from build123d import *

# Parameters (mm, degrees)
SKETCH_1_W             = 40
SKETCH_1_H             = 27
EXTRUDE_1_DEPTH        = 60
SKETCH_2_R             = 2.5
CUT_EXTRUDE_1_DEPTH    = 27
PATTERN_LINEAR_1_COUNT = 2
PATTERN_LINEAR_1_PITCH = 46
SKETCH_4_R             = 1.65
CUT_EXTRUDE_3_DEPTH    = 27
SKETCH_5_W             = 20
SKETCH_5_H             = 60
CUT_EXTRUDE_4_DEPTH    = 30
PATTERN_LINEAR_2_COUNT = 2
PATTERN_LINEAR_2_PITCH = 10


with BuildPart() as part:
    # Эскиз1 → Бобышка-Вытянуть1 (new body)
    with BuildSketch(Plane.XY):
        Rectangle(SKETCH_1_W, SKETCH_1_H)
    extrude(amount=EXTRUDE_1_DEPTH)

    # Эскиз2 → Вырез-Вытянуть1 (cut)
    with BuildSketch(Plane(origin=(0, 13.5, 0), x_dir=(1, 0, 0), z_dir=(0, 1, 0))):
        with Locations(Location((-10, -7, 0), (0, 0, 180))):
            Circle(SKETCH_2_R)
    cut_extrude_1 = extrude(amount=-CUT_EXTRUDE_1_DEPTH, mode=Mode.SUBTRACT)

    # Линейный массив1: Вырез-Вытянуть1 ×2
    with Locations(*[(0, 0, i * PATTERN_LINEAR_1_PITCH) for i in range(1, PATTERN_LINEAR_1_COUNT)]):
        add(cut_extrude_1, mode=Mode.SUBTRACT)

    # Эскиз4 → Вырез-Вытянуть3 (cut)
    with BuildSketch(Plane(origin=(0, 13.5, 0), x_dir=(1, 0, 0), z_dir=(0, 1, 0))):
        with Locations(Location((-15, -15, 0), (0, 0, 270))):
            Circle(SKETCH_4_R)
        with Locations(Location((-15, -45, 0), (0, 0, 270))):
            Circle(SKETCH_4_R)
    cut_extrude_3 = extrude(amount=-CUT_EXTRUDE_3_DEPTH, mode=Mode.SUBTRACT)

    # Эскиз5 → Вырез-Вытянуть4 (cut)
    with BuildSketch(Plane.XZ.offset(13.5)):
        with Locations((10, 30)):
            Rectangle(SKETCH_5_W, SKETCH_5_H)
    extrude(amount=-CUT_EXTRUDE_4_DEPTH, mode=Mode.SUBTRACT)

    # Линейный массив2: Вырез-Вытянуть3 ×2
    with Locations(*[(i * PATTERN_LINEAR_2_PITCH, 0, 0) for i in range(1, PATTERN_LINEAR_2_COUNT)]):
        add(cut_extrude_3, mode=Mode.SUBTRACT)


solid = part.part
Input: part model. Units: mm. Frame: model coordinates. Round coordinates to 2 decimals unless told otherwise and drop trailing zeros. Loops run counter-clockwise (first coordinate to the right, second up) from the corner with the lowest first, then second, coordinate; pieces in that order, holes last. Notation, with made-up numbers: (60.5, 80) -> (106.5, 80) arc R19 cw to (106.5, 110) -> close; hole circle Ø11 at (18.5, -7.5). An arc over 180 degrees is marked (long way). Answer as a JSON object with one key per item and string values. Group by question number.
1) Pin query (flat end, axial travel): pin 1 (3 mm diameter, centred on y = -8, z = 12, fed in from +X). Return the tip coordinate at first contact, or that it passes through.
2) Section query A-A on x = -10. Output: boundary loops of the cut face in (y, z).
3) Section query D-D on z = 45. Output: boundary loops of the cut face in (x, y).
4) Section query B-B on y = -5. Output: boundary loops of the cut face in (x, z), plus the area to 3 significant figures.
5) Ray query, L1, parallel to Z at x = -10, y = 7.5; L2, parallel to X at y = -1.5, z = 15; L3, parallel to Z at x = -5.75, y = -2.5. Return the intervals inside material, ascending.
6) Draft query along X for faces 1 (the flat face through (-10, 0, 0)), 2 (the cylindrical face through (-9.67, 0.19, 55.48)), 3 (the flat face through (-20, 0, 30)), 4 (the flat face through (0, 0, 30)). Return one class per face: +X half, -X half, draft (parallel to the pull), parting line (faces both ways), or undercut.
7) Section query C-C on z = 53. Output: boundary loops of the cut face in (x, y).
Reply:
{
 "1": {"pin 1": "stops at x = 0"},
 "2": {"outline": "(-13.5, 0) -> (13.5, 0) -> (13.5, 4.5) -> (-13.5, 4.5) -> close; (-13.5, 9.5) -> (13.5, 9.5) -> (13.5, 50.5) -> (-13.5, 50.5) -> close; (-13.5, 55.5) -> (13.5, 55.5) -> (13.5, 60) -> (-13.5, 60) -> close"},
 "3": {"outline": "(-20, -13.5) -> (-16.65, -13.5) -> (-16.65, 13.5) -> (-20, 13.5) -> close; (-13.35, -13.5) -> (-6.65, -13.5) -> (-6.65, 13.5) -> (-13.35, 13.5) -> close; (-3.35, -13.5) -> (0, -13.5) -> (0, 13.5) -> (-3.35, 13.5) -> close"},
 "4": {"outline": "(-20, 0) -> (0, 0) -> (0, 60) -> (-20, 60) -> close; hole circle Ø3.3 at (-15, 15); hole circle Ø3.3 at (-15, 45); hole circle Ø5 at (-10, 7); hole circle Ø5 at (-10, 53); hole circle Ø3.3 at (-5, 15); hole circle Ø3.3 at (-5, 45)", "area": "1,130 mm2"},
 "5": {"L1": "z = 0 to 4.5, 9.5 to 50.5, 55.5 to 60", "L2": "x = -20 to -16.65, -13.35 to -6.65, -3.35 to 0", "L3": "z = 0 to 13.53, 16.47 to 43.53, 46.47 to 60"},
 "6": {"face 1": "draft", "face 2": "undercut", "face 3": "-X half", "face 4": "+X half"},
 "7": {"outline": "(-20, -13.5) -> (-12.5, -13.5) -> (-12.5, 13.5) -> (-20, 13.5) -> close; (-7.5, -13.5) -> (0, -13.5) -> (0, 13.5) -> (-7.5, 13.5) -> close"}
}
